Autodesk Inventor part; units mm, degrees
ref_plane "YZ Plane" through (0, 0, 0) normal (1, 0, 0) x (0, 1, 0)
ref_plane "XZ Plane" through (0, 0, 0) normal (0, 1, 0) x (-1, 0, 0)
ref_plane "XY Plane" through (0, 0, 0) normal (0, 0, 1) x (1, 0, 0)
sketch "Sketch1" plane through (0, 0, 0) normal (0, 1, 0) x (-1, 0, 0)
  line L0 (1839.667, -285.297) -> (163.267, -285.297)
  line L1 (163.267, -285.297) -> (163.267, -590.097)
  line L2 (163.267, -590.097) -> (1839.667, -590.097)
  arc A0 (1839.667, -590.097) -> (1839.667, -285.297) centre (1839.667, -437.697) ccw
  line L3 (1839.667, -590.097) -> (1839.667, -285.297) construction
  point P0 (0, 0)
  dimension "d0" = 1828.8
  dimension "d2" = 152.4
  dimension "d5" = 304.8
  dimension "d43" = 590.097
  dimension "d59" = 1839.667
extrude "Extrusion1" add sketch "Sketch1" along normal blind 254
shell "Shell1" thickness 17.8562 removed faces 0
sketch "Sketch2" plane through (-163.267, 0, -590.097) normal (0, 0, -1) x (-1, 0, 0)
  circle A0 centre (355.6, 158.75) radius 73.025
  line L0 (0, 0) -> (0, 254)
  line L1 (0, 254) -> (1676.4, 254)
  circle A1 centre (558.8, 158.75) radius 73.025
  circle A2 centre (762, 158.75) radius 73.025
  circle A3 centre (965.2, 158.75) radius 73.025
  circle A4 centre (1168.4, 158.75) radius 73.025
  circle A5 centre (1371.6, 158.75) radius 73.025
  circle A6 centre (1574.8, 158.75) radius 73.025
  circle A7 centre (304.8, 44.45) radius 25.4
  circle A8 centre (406.4, 44.45) radius 25.4
  circle A9 centre (508, 44.45) radius 25.4
  circle A10 centre (609.6, 44.45) radius 25.4
  circle A11 centre (711.2, 44.45) radius 25.4
  circle A12 centre (812.8, 44.45) radius 25.4
  circle A13 centre (914.4, 44.45) radius 25.4
  circle A14 centre (1016, 44.45) radius 25.4
  circle A15 centre (1117.6, 44.45) radius 25.4
  circle A16 centre (1219.2, 44.45) radius 25.4
  circle A17 centre (1320.8, 44.45) radius 25.4
  circle A18 centre (1422.4, 44.45) radius 25.4
  circle A19 centre (1524, 44.45) radius 25.4
  circle A20 centre (1625.6, 44.45) radius 25.4
  point P0 (-163.267, 0)
  dimension "d11" = 146.05
  dimension "d12" = 355.6
  dimension "d13" = 95.25
  dimension "d19" = 203.2
  dimension "d21" = 304.8
  dimension "d22" = 209.55
  dimension "d23" = 50.8
  dimension "d26" = 101.6
extrude "Extrusion4" cut sketch "Sketch2" against normal blind 50.8
sketch "Sketch9" plane through (-163.267, 0, -285.297) normal (1, 0, 0) x (0, 0, -1)
  line L0 (406.4, -101.6) -> (-101.6, -101.6)
  line L1 (-152.4, -50.8) -> (-152.4, 304.8)
  line L2 (-101.6, 355.6) -> (406.4, 355.6)
  line L3 (457.2, 304.8) -> (457.2, -50.8)
  line L4 (304.8, 0) -> (0, 0) construction
  line L5 (152.4, 0) -> (152.4, -101.6) construction
  line L6 (304.8, 0) -> (304.8, 254) construction
  line L7 (304.8, 127) -> (457.2, 127) construction
  arc A0 (406.4, -101.6) -> (457.2, -50.8) centre (406.4, -50.8) ccw
  arc A1 (-152.4, -50.8) -> (-101.6, -101.6) centre (-101.6, -50.8) ccw
  arc A2 (-101.6, 355.6) -> (-152.4, 304.8) centre (-101.6, 304.8) ccw
  arc A3 (457.2, 304.8) -> (406.4, 355.6) centre (406.4, 304.8) ccw
  point P0 (-285.297, 0)
  point P1 (457.2, -101.6)
  point P2 (-152.4, -101.6)
  point P3 (457.2, 355.6)
  dimension "d50" = 457.2
  dimension "d51" = 609.6
  dimension "d52" = 50.8
extrude "Extrusion5" add sketch "Sketch9" along normal blind 37.084
sketch "Sketch10" plane through (-1839.667, 0, -590.097) normal (0, 0, -1) x (-1, 0, 0)
  line L0 (-406.4, 751.6147) -> (-406.4, -779.9775) construction
  line L1 (-1676.4, 304.8) -> (-1676.4, -50.8) construction
  point P0 (-1839.667, 0)
  dimension "d55" = 1531.5921
  dimension "d56" = 1270
sketch "Sketch11" plane through (0, 254, 0) normal (0, 1, 0) x (1, 0, 0)
  line L0 (-1839.667, 285.297) -> (-1839.667, 590.097)
  line L1 (-1839.667, 590.097) -> (-1821.125, 590.097)
  line L2 (-163.267, 590.097) -> (-1839.667, 590.097)
  arc A0 (-1839.667, 590.097) -> (-1839.667, 285.297) centre (-1839.667, 437.697) ccw
  line L3 (-1821.887, 285.297) -> (-1839.667, 285.297)
  line L4 (-1821.887, 285.297) -> (-1821.887, 590.097)
  line L5 (-1821.887, 590.097) -> (-1839.667, 590.097)
  point P0 (0, 0)
  dimension "d58" = 17.78
extrude "Extrusion6" add sketch "Sketch11" against normal blind 254 contours L0 L1 L4 L3
sketch "Sketch12" plane through (-1821.887, 17.8562, -303.1532) normal (1, 0, 0) x (0, 0, -1)
  line L0 (269.0876, 218.2876) -> (0, 218.2876)
  line L1 (198.0438, 218.2876) -> (198.0438, 0)
  line L2 (0, 0) -> (269.0876, 0)
  line L3 (198.0438, 0) -> (180.2638, 0)
  line L4 (180.2638, 0) -> (180.2638, 218.2876)
  line L5 (180.2638, 218.2876) -> (198.0438, 218.2876)
  line L6 (286.9438, -17.8562) -> (286.9438, 236.1438)
  point P0 (-303.1532, -17.8562)
  dimension "d62" = 17.78
  dimension "d63" = 88.9
extrude "Extrusion7" add sketch "Sketch12" along normal blind 1651
properties part number "LineArray"
For this review, take the finished solid that the model builds, in its own axes (mm). A direction names the side the tool comes from. Coordinates: 2 decimals unless noted, no trailing zeros. Order: outer loops, then holes, each group sorted by start corner. A loop starts at its lowest first (then second) coordinate and runs counter-clockwise, first axis right, second up. Notation, with made-up numbers: (17, -27) - (28, -27) arc R12 cw to (28, -17) - close; hole circle Ø2 at (81.5, 20). An arc over 180 degrees is marked (long way). Answer as CSV lines item,"result". Start each with the question number.
1) Add section B-B (z = -384). State the section outline as (x, y) points.
2) Insertion check: P1, Ø8, axis at y = 244, z = -569.5, coming from the -X side; P2, Ø1.5, axis at x = -914, z = -365.5, coming from the -Y side; P3, Ø3, axis at y = 148, z = -372.5, coming from the -X side. Each pin has a flat end and moves straight along its axis. Give the tip position at first contact, or say it passes through.
3) Draft analysis for pull direction Y (two halves, no side actions). For faces 4 (the cylindrical face through (-1992.03, 125.22, -434.35)), 5 (the cylindrical face through (-1258.713, 161.961, -581.294)), state which applies: +Y half, -Y half, draft (parallel to the pull), parting line (faces both ways), or undercut.
4) Add section C-C (y = 44.45). Count the separate pieces of the cut face and the enclosed holes in it, then the cut area to 3 significant figures.
5) Machinability: for faces 1 (the cylindrical face through (-1665.113, 161.961, -581.294)), 2 (the flat face through (-803, 125, -590.097)), 3 (the flat face through (-990, 236.144, -536)), which of the approach directions +Z, -Z, +X, -X, +Y, -Y give a long, thin tool a straight path to every point of the face, cutting with its end or side? Answer none if there is none.
6) To check wall thickness, follow line 1 along Z through (x, y) = (-452, 92); line 2 along Y through (x, z) = (-1169.5, -450.5); line 3 along Z through (x, y) = (-1369, 45). State the ranges of each line that lie inside material, in increasing order. Write a range as [from, to].
7) Add section A-A (x = -263). State the section outline as (y, z) points.
Result:
1,outline,"(-1982.29, 0) - (-163.27, 0) - (-163.27, -101.6) - (-126.18, -101.6) - (-126.18, 355.6) - (-163.27, 355.6) - (-163.27, 254) - (-1982.29, 254) - close; hole (-1963.03, 17.86) - (-1839.67, 17.86) - (-1839.67, 236.14) - (-1963.03, 236.14) - close; hole (-1821.89, 17.86) - (-181.12, 17.86) - (-181.12, 236.14) - (-1821.89, 236.14) - close"
2,P1,"x = -1922.69"
2,P2,"y = 0"
2,P3,"x = -1978.12"
3,face 4,"draft"
3,face 5,"undercut"
4,separate pieces,"14"
4,enclosed holes,"2"
4,area,"117,000 mm^2"
5,face 1,"-Z"
5,face 2,"-Z, -X, +Y, -Y"
5,face 3,"none"
6,line 1,"[-590.1, -572.24], [-501.2, -483.42], [-303.15, -285.3]"
6,line 2,"[0, 17.86], [236.14, 254]"
6,line 3,"[-501.2, -483.42], [-303.15, -285.3]"
7,outline,"(0, -590.1) - (254, -590.1) - (254, -285.3) - (0, -285.3) - close; hole (17.86, -572.24) - (236.14, -572.24) - (236.14, -501.2) - (17.86, -501.2) - close; hole (17.86, -483.42) - (236.14, -483.42) - (236.14, -303.15) - (17.86, -303.15) - close"
